Design review of the part shown in the three views and the two pictorial views. Dimensions are in mm from the part's minimum x, y and z. A direction names the side the tool comes from. Coordinates: 2 decimals unless noted, no trailing zeros. Order: outer loops, then holes, each group sorted by start corner. A loop starts at its lowest first (then second) coordinate and runs counter-clockwise, first axis right, second up. Notation, with made-up numbers: (3.5, 8.25) - (23.5, 8.25) arc R33 ccw to (23.5, 37.25) - close; hole circle Ø10 at (82, 73.5). An arc over 180 degrees is marked (long way). One line per item, written item: value. Start each with the question number.
(1) Consider section D-D on z = 2. Write out the cut boundary in (x, y).
(2) Mouldability with a two-part tool opening along Z and no side actions: class the marked faces 1, 2 and 3 as released by +Z, released by -Z, zero draft, split by the parting line, or undercut.
(3) Consider section C-C on y = 8. Write out the cut boundary in (x, z), then the cut area to 3 significant figures.
(4) For the marked faces 4 and 5, list the 3-axis set-ups (+Z, -Z, +X, -X, +Y, -Y) from which the entire face can be reached by the end or side of a thin tool; tool diameter is ignored.
(5) Clearance check with flat-ended pins moving along their axes: pin 1 (2.5 mm diameter, centred on x = 3, z = 11, fed in from -Y); pin 2 (6 mm diameter, centred on x = 17.5, z = 18, fed in from +Y); pin 3 (5 mm diameter, centred on x = 11, y = 8, fed in from +Z); pin 4 (4 mm diameter, centred on y = 5.5, z = 8, fed in from +X). State where each tip first meets the part, or that it passes through.
(6) Consider section B-B on z = 11. Write out the cut boundary in (x, y).
(7) Consider section A-A on x = 11. Write out the cut boundary in (y, z), then the cut area to 3 significant figures.
(8) To check wall thickness, follow line 1 along X through (y, z) = (6, 11); line 2 along Y through (x, z) = (11, 14.8); line 3 along Y through (x, z) = (17, 14.5). State the ranges of each line that lie inside material, in increasing order.
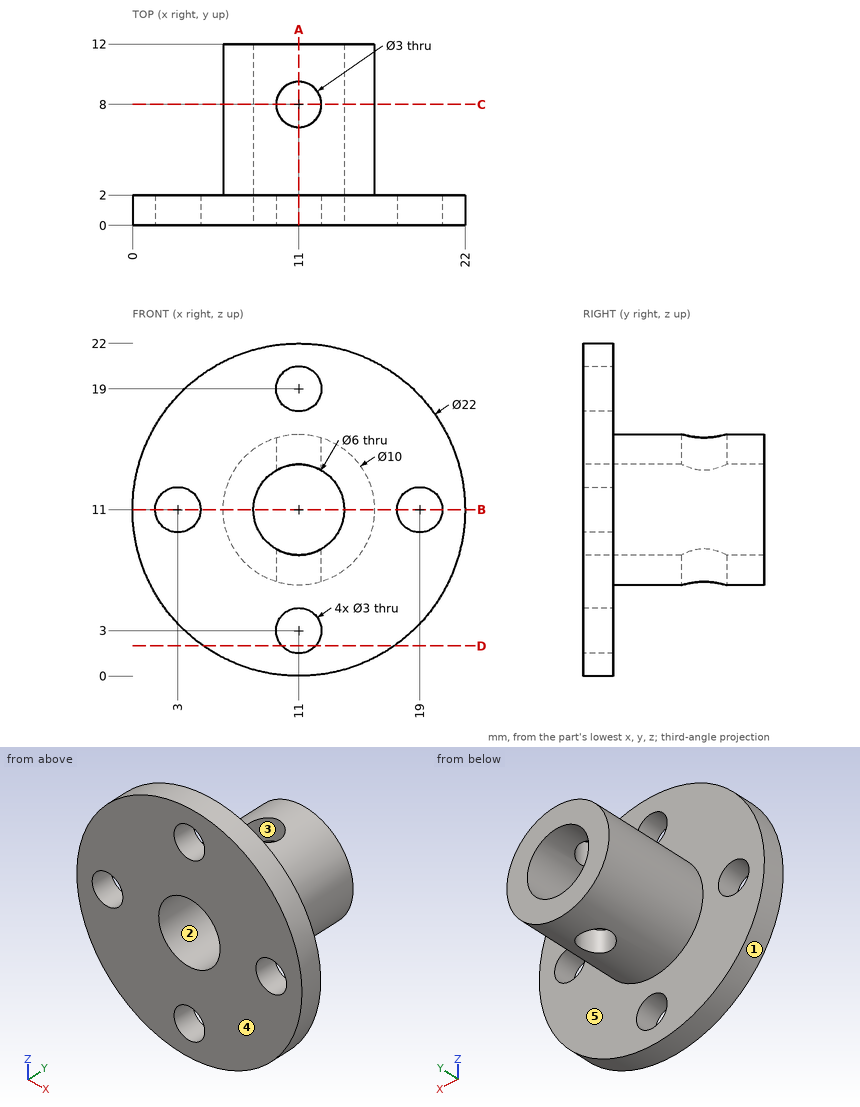
Geometry check:
1. outline: (4.68, 0) - (9.88, 0) - (9.88, 2) - (4.68, 2) - close; (12.12, 0) - (17.32, 0) - (17.32, 2) - (12.12, 2) - close
2. face 1: split by the parting line
2. face 2: undercut
2. face 3: zero draft
3. outline: (9.5, 6.23) - (9.5, 8.4) arc R3 cw to (9.5, 13.6) - (9.5, 15.77) arc R5 ccw to start; (12.5, 6.23) arc R5 ccw to (12.5, 15.77) - (12.5, 13.6) arc R3 cw to (12.5, 8.4) - close
3. area: 37.9 mm^2
4. face 4: +Z, -Z, +X, -X, -Y
4. face 5: +Y
5. pin 1: passes through
5. pin 2: stops at y = 2
5. pin 3: stops at z = 16
5. pin 4: stops at x = 15.9
6. outline: (0, 0) - (1.5, 0) - (1.5, 2) - (0, 2) - close; (4.5, 0) - (8, 0) - (8, 12) - (6, 12) - (6, 2) - (4.5, 2) - close; (14, 0) - (17.5, 0) - (17.5, 2) - (16, 2) - (16, 12) - (14, 12) - close; (20.5, 0) - (22, 0) - (22, 2) - (20.5, 2) - close
7. outline: (0, 0) - (2, 0) - (2, 1.5) - (0, 1.5) - close; (0, 4.5) - (2, 4.5) - (2, 6) - (6.5, 6) - (6.5, 8) - (0, 8) - close; (0, 14) - (6.5, 14) - (6.5, 16) - (2, 16) - (2, 17.5) - (0, 17.5) - close; (0, 20.5) - (2, 20.5) - (2, 22) - (0, 22) - close; (9.5, 6) - (12, 6) - (12, 8) - (9.5, 8) - close; (9.5, 14) - (12, 14) - (12, 16) - (9.5, 16) - close
7. area: 48.0 mm^2
8. line 1: x = 6 to 8, 14 to 16
8. line 2: y = 0 to 6.5, 9.5 to 12
8. line 3: y = 0 to 2
